from build123d import *

# Parameters (mm, degrees)
SKETCH_1_W            = 113
SKETCH_1_H            = 83
EXTRUDE_1_DEPTH       = 24
SKETCH_21_W           = 113
SKETCH_21_H           = 2
EXTRUDE_2_DEPTH       = 52.5
CUT_EXTRUDE_20_DEPTH  = 25
MIRROR_2_COPY_1_DEPTH = 25
SKETCH_27_R           = 4
EXTRUDE_4_DEPTH       = 10
SKETCH_28_R           = 0.835314329
SKETCH_28_R_2         = 0.866649433
EXTRUDE_5_DEPTH       = 10


with BuildPart() as part:
    # Sketch 1 → Extrude 1 (new body)
    with BuildSketch(Plane(origin=(0, 31, 0), x_dir=(1, 0, 0), z_dir=(0, 1, 0))):
        Rectangle(SKETCH_1_W, SKETCH_1_H)
    extrude(amount=-EXTRUDE_1_DEPTH)

    # Sketch 21 → Extrude 2 (add, symmetric)
    with BuildSketch(Plane(origin=(0, 0, 0), x_dir=(-1, 0, 0), z_dir=(0, 0, -1))):
        with Locations((0, 30)):
            Rectangle(SKETCH_21_W, SKETCH_21_H)
    extrude(amount=EXTRUDE_2_DEPTH, both=True)

    # Sketch 22 → Cut-Extrude 20 (cut, through all)
    with BuildSketch(Plane(origin=(0, 31, 0), x_dir=(-1, 0, 0), z_dir=(0, 1, 0))):
        with BuildLine():
            Line((-26.5, -49.5), (-33.5, -49.5))
            ThreePointArc((-33.5, -49.5), (-36, -47), (-33.5, -44.5))
            Line((-33.5, -44.5), (-26.5, -44.5))
            ThreePointArc((-26.5, -44.5), (-24, -47), (-26.5, -49.5))
        make_face()
    cut_extrude_20 = extrude(amount=-CUT_EXTRUDE_20_DEPTH, mode=Mode.SUBTRACT)

    # Mirror 1: Cut-Extrude 20 across plane
    add(cut_extrude_20.mirror(Plane(origin=(0, 0, 0), x_dir=(0, 0, 1), z_dir=(1, 0, 0))), mode=Mode.SUBTRACT)

    # Mirror 2: Cut-Extrude 20 across plane
    add(cut_extrude_20.mirror(Plane.XY), mode=Mode.SUBTRACT)

    # Mirror 2 copy 1 sketch → Mirror 2 copy 1 (cut, through all)
    with BuildSketch(Plane(origin=(0, 31, 0), x_dir=(1, 0, 0), z_dir=(0, 1, 0))):
        with BuildLine():
            Line((-26.5, -49.5), (-33.5, -49.5))
            ThreePointArc((-33.5, -49.5), (-36, -47), (-33.5, -44.5))
            Line((-33.5, -44.5), (-26.5, -44.5))
            ThreePointArc((-26.5, -44.5), (-24, -47), (-26.5, -49.5))
        make_face()
    extrude(amount=-MIRROR_2_COPY_1_DEPTH, mode=Mode.SUBTRACT)

    # Sketch 27 → Extrude 4 (add)
    with BuildSketch(Plane.ZY.offset(56.5)):
        with Locations((0, 19)):
            Circle(SKETCH_27_R)
    extrude_4 = extrude(amount=EXTRUDE_4_DEPTH)

    # Mirror 3: Extrude 4 across plane
    add(extrude_4.mirror(Plane(origin=(0, 0, 0), x_dir=(0, 0, 1), z_dir=(1, 0, 0))))

    # Sketch 28 → Extrude 5 (add)
    with BuildSketch(Plane(origin=(56.5, 0, 0), x_dir=(0, 0, -1), z_dir=(1, 0, 0))):
        with Locations((26.586559597, 18.769220483)):
            Circle(SKETCH_28_R)
        with Locations((33.466100625, 18.769220483)):
            Circle(SKETCH_28_R_2)
    extrude(amount=EXTRUDE_5_DEPTH)


solid = part.part
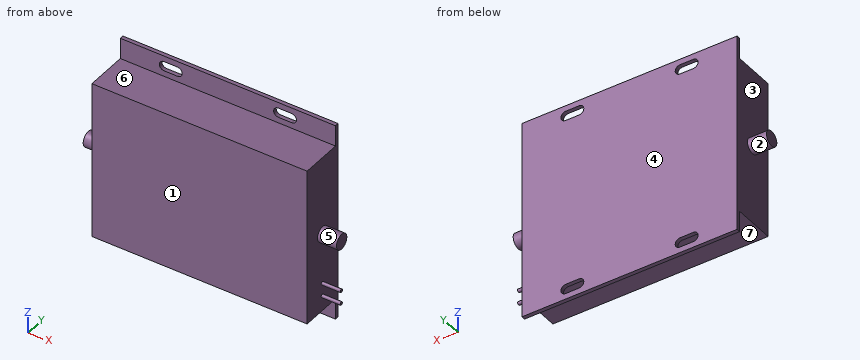
Read the model definition and answer for the solid it produces. Units are mm, in the model's axes. Face numbers are marked on the shaded views. A direction names the side the tool comes from. Give positions to 0.01 mm unless a question says otherwise; leave off trailing zeros. Write each loop counter-clockwise with the first axis right and the second up, starting at its lowest first coordinate (ties: lowest second). Pieces come first, ordered by that corner, then holes. Notation, with made-up numbers: (39.5, -35.75) - (97.5, -35.75) arc R20 cw to (97.5, -18.75) - close; hole circle Ø7 at (58, -12). An arc over 180 degrees is marked (long way). Return JSON: item names as keys, results as strings.
Q1. A cutting plane is placed at A-A, the plane z = 47. Determine the outline of the cut face in (x, y).
Reply:
{"outline": "(-56.5, 29) - (-36, 29) - (-36, 31) - (-56.5, 31) - close; (-24, 29) - (24, 29) - (24, 31) - (-24, 31) - close; (36, 29) - (56.5, 29) - (56.5, 31) - (36, 31) - close"}
Q2. A cutting plane is placed at B-B, the plane z = 0. Determine the outline of the cut face in (x, y), and give its area (3 significant figures).
Reply:
{"outline": "(-66.5, 15) - (-56.5, 15) - (-56.5, 7) - (56.5, 7) - (56.5, 15) - (66.5, 15) - (66.5, 23) - (56.5, 23) - (56.5, 31) - (-56.5, 31) - (-56.5, 23) - (-66.5, 23) - close", "area": "2,870 mm²"}
Q3. Consider line 1 along X through (y, z) = (29, -21.5); line 2 along Z through (x, y) = (6, 26.5); line 3 along Y through (x, z) = (50.5, -42.5). Determine where each line is inside the solid, lowest interval first. Write a range as [from, to].
Reply:
{"line 1": "[-56.5, 56.5]", "line 2": "[-41.5, 41.5]", "line 3": "[29, 31]"}
Q4. A cutting plane is placed at C-C, the plane x = -6.5. Determine the outline of the cut face in (y, z), and give its area (3 significant figures).
Reply:
{"outline": "(7, -41.5) - (29, -41.5) - (29, -52.5) - (31, -52.5) - (31, 52.5) - (29, 52.5) - (29, 41.5) - (7, 41.5) - close", "area": "2,040 mm²"}
Q5. For the marked faces 5, 6 and 7, determine the directions among +Z, -Z, +X, -X, +Y, -Y from which every point of the face is accessible in a straight line to the end or side of a thin tool.
Reply:
{"face 5": "+X", "face 6": "+Z, +X, -X, -Y", "face 7": "-Z, +X, -X, -Y"}
Q6. Given P1, Ø10, axis at y = 17, z = -28, coming from the -X side; P2, Ø6, axis at x = -49, y = 14.5, coming from the -Z side; P3, Ø1, axis at x = -10.5, y = 14.5, coming from the +Z side, each flat-ended and moving along its own axis, determine where each tip first touches the part or whether it passes through.
Reply:
{"P1": "x = -56.5", "P2": "z = -41.5", "P3": "z = 41.5"}
Q7. For a pull along Y with two mould halves and no side action, classify the marked faces 1, 2, 3 and 4 as released by +Y, released by -Y, zero draft, split by the parting line, or undercut.
Reply:
{"face 1": "released by -Y", "face 2": "split by the parting line", "face 3": "zero draft", "face 4": "released by +Y"}
Q8. A cutting plane is placed at D-D, the plane y = 25.75. Determine the outline of the cut face in (x, z).
Reply:
{"outline": "(-56.5, -41.5) - (56.5, -41.5) - (56.5, 41.5) - (-56.5, 41.5) - close"}
